Here's how the part is built. I have some questions about the finished solid (model axes, mm). Face numbers are marked on the shaded views. A direction names the side the tool comes from. Give positions to 0.01 mm unless a question says otherwise; leave off trailing zeros. Loops run counter-clockwise (first coordinate to the right, second up) from the corner with the lowest first, then second, coordinate; pieces in that order, holes last.
Q1. Suppose I cut it at A-A (x = 0). List the corners of the cut face in (y, z) for me.
Q2. For the marked faces 1 and 2, which set-ups out of +Z, -Z, +X, -X, +Y, -Y let a thin tool reach every point of the face, with its end or its side?
Q3. I need wall thicknesses on probe 1 along Y at (x, z) = (-10.5, 215); probe 2 along Y at (x, z) = (0, 220.5). Which ranges of each line are inside material? Lowest first, please.
Q4. Thinking about a two-plate mould opening in X: for the marked faces 3, 4, 5 and 6, which applies, pulls with the +X half, pulls with the -X half, needs draft (parallel to the pull), parting line crosses it, or undercut?
Q5. Suppose I cut it at B-B (y = -11.75). List the corners of the cut face in (x, z) for me, and give its area (3 significant figures).
Q6. I'm going to push flat-ended pins straight in: P1, Ø4.5, axis at y = -1, z = 220.5, coming from the +X side; P2, Ø0.7, axis at x = -4.5, z = 214.5, coming from the -Y side; P3, Ø0.6, axis at y = 14.5, z = 228.5, coming from the -X side. Where does each tip first touch, or does it pass through?
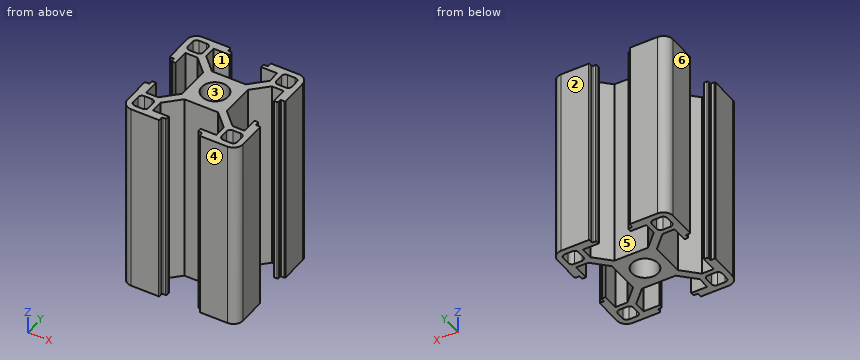
```python
from build123d import *

# Parameters (mm, degrees)
BOSS_EXTRUDE1_DEPTH = 250
SKETCH2_R           = 3.4
CUT_EXTRUDE1_DEPTH  = 251.898385806
FILLET1_R           = 2.5
FILLET2_R           = 0.25
CUT_EXTRUDE3_START  = -200
SKETCH3_R           = 3.4
CUT_EXTRUDE3_DEPTH  = 200


with BuildPart() as part:
    # Sketch1 → Boss-Extrude1 (new body)
    with BuildSketch(Plane.XY):
        Polygon((-15, 15), (-5.2, 15), (-5.2, 13.808325472), (-4.1, 13.808325472), (-4.1, 12.8), (-8.25, 12.8), (-8.25, 9.664213562), (-4.385786438, 5.8), (4.385786438, 5.8), (8.25, 9.664213562), (8.25, 12.8), (4.1, 12.8), (4.1, 13.808325472), (5.2, 13.808325472), (5.2, 15), (15, 15), (15, 5.2), (13.808325472, 5.2), (13.808325472, 4.1), (12.8, 4.1), (12.8, 8.25), (9.664213562, 8.25), (5.8, 4.385786438), (5.8, -4.385786438), (9.664213562, -8.25), (12.8, -8.25), (12.8, -4.1), (13.808325472, -4.1), (13.808325472, -5.2), (15, -5.2), (15, -15), (5.2, -15), (5.2, -13.808325472), (4.1, -13.808325472), (4.1, -12.8), (8.25, -12.8), (8.25, -9.664213562), (4.385786438, -5.8), (-4.385786438, -5.8), (-8.25, -9.664213562), (-8.25, -12.8), (-4.1, -12.8), (-4.1, -13.808325472), (-5.2, -13.808325472), (-5.2, -15), (-15, -15), (-15, -5.2), (-13.808325472, -5.2), (-13.808325472, -4.1), (-12.8, -4.1), (-12.8, -8.25), (-9.664213562, -8.25), (-5.8, -4.385786438), (-5.8, 4.385786438), (-9.664213562, 8.25), (-12.8, 8.25), (-12.8, 4.1), (-13.808325472, 4.1), (-13.808325472, 5.2), (-15, 5.2), align=None)
    extrude(amount=BOSS_EXTRUDE1_DEPTH)

    # Sketch2 → Cut-Extrude1 (cut, through all)
    with BuildSketch(Plane.XY.offset(250)):
        Circle(SKETCH2_R)
        with BuildLine():
            Line((-12.5, 13.5), (-10.5, 13.5))
            ThreePointArc((-10.5, 13.5), (-9.792893219, 13.207106781), (-9.5, 12.5))
            Line((-9.5, 12.5), (-9.5, 10.5))
            ThreePointArc((-9.5, 10.5), (-9.792893219, 9.792893219), (-10.5, 9.5))
            Line((-10.5, 9.5), (-12.5, 9.5))
            ThreePointArc((-12.5, 9.5), (-13.207106781, 9.792893219), (-13.5, 10.5))
            Line((-13.5, 10.5), (-13.5, 12.5))
            ThreePointArc((-13.5, 12.5), (-13.207106781, 13.207106781), (-12.5, 13.5))
        make_face()
        with BuildLine():
            Line((9.5, 12.5), (9.5, 10.5))
            ThreePointArc((9.5, 10.5), (9.792893219, 9.792893219), (10.5, 9.5))
            Line((10.5, 9.5), (12.5, 9.5))
            ThreePointArc((12.5, 9.5), (13.207106781, 9.792893219), (13.5, 10.5))
            Line((13.5, 10.5), (13.5, 12.5))
            ThreePointArc((13.5, 12.5), (13.207106781, 13.207106781), (12.5, 13.5))
            Line((12.5, 13.5), (10.5, 13.5))
            ThreePointArc((10.5, 13.5), (9.792893219, 13.207106781), (9.5, 12.5))
        make_face()
        with BuildLine():
            Line((12.5, -13.5), (10.5, -13.5))
            ThreePointArc((10.5, -13.5), (9.792893219, -13.207106781), (9.5, -12.5))
            Line((9.5, -12.5), (9.5, -10.5))
            ThreePointArc((9.5, -10.5), (9.792893219, -9.792893219), (10.5, -9.5))
            Line((10.5, -9.5), (12.5, -9.5))
            ThreePointArc((12.5, -9.5), (13.207106781, -9.792893219), (13.5, -10.5))
            Line((13.5, -10.5), (13.5, -12.5))
            ThreePointArc((13.5, -12.5), (13.207106781, -13.207106781), (12.5, -13.5))
        make_face()
        with BuildLine():
            Line((-9.5, -12.5), (-9.5, -10.5))
            ThreePointArc((-9.5, -10.5), (-9.792893219, -9.792893219), (-10.5, -9.5))
            Line((-10.5, -9.5), (-12.5, -9.5))
            ThreePointArc((-12.5, -9.5), (-13.207106781, -9.792893219), (-13.5, -10.5))
            Line((-13.5, -10.5), (-13.5, -12.5))
            ThreePointArc((-13.5, -12.5), (-13.207106781, -13.207106781), (-12.5, -13.5))
            Line((-12.5, -13.5), (-10.5, -13.5))
            ThreePointArc((-10.5, -13.5), (-9.792893219, -13.207106781), (-9.5, -12.5))
        make_face()
    extrude(amount=-CUT_EXTRUDE1_DEPTH, mode=Mode.SUBTRACT)

    # Fillet1
    fillet1_edges = [part.edges().sort_by_distance(p)[0] for p in [
        (15, -15, 125),
        (-15, -15, 125),
        (-15, 15, 125),
        (15, 15, 125),
    ]]
    fillet(fillet1_edges, radius=FILLET1_R)

    # Fillet2
    fillet2_edges = [part.edges().sort_by_distance(p)[0] for p in [
        (5.2, -15, 125),
        (5.2, -13.808325472, 125),
        (4.1, -13.808325472, 125),
        (-4.1, -13.808325472, 125),
        (-5.2, -13.808325472, 125),
        (-5.2, -15, 125),
        (-15, -5.2, 125),
        (-13.808325472, -5.2, 125),
        (-13.808325472, -4.1, 125),
        (-13.808325472, 4.1, 125),
        (-13.808325472, 5.2, 125),
        (-15, 5.2, 125),
        (-5.2, 15, 125),
        (-5.2, 13.808325472, 125),
        (-4.1, 13.808325472, 125),
        (4.1, 13.808325472, 125),
        (5.2, 13.808325472, 125),
        (5.2, 15, 125),
        (15, 5.2, 125),
        (13.808325472, 5.2, 125),
        (13.808325472, 4.1, 125),
        (13.808325472, -4.1, 125),
        (13.808325472, -5.2, 125),
        (15, -5.2, 125),
    ]]
    fillet(fillet2_edges, radius=FILLET2_R)

    # Sketch3 → Cut-Extrude3 (cut)
    with BuildSketch(Plane(origin=(0, 0, 0), x_dir=(-1, 0, 0), z_dir=(0, 0, -1)).offset(CUT_EXTRUDE3_START)):
        with BuildLine():
            Line((12.8, 4.1), (13.558325472, 4.1))
            ThreePointArc((13.558325472, 4.1), (13.735102167, 4.173223305), (13.808325472, 4.35))
            Line((13.808325472, 4.35), (13.808325472, 4.95))
            ThreePointArc((13.808325472, 4.95), (13.881548777, 5.126776695), (14.058325472, 5.2))
            Line((14.058325472, 5.2), (14.75, 5.2))
            ThreePointArc((14.75, 5.2), (14.926776695, 5.273223305), (15, 5.45))
            Line((15, 5.45), (15, 12.5))
            ThreePointArc((15, 12.5), (14.267766953, 14.267766953), (12.5, 15))
            Line((12.5, 15), (5.45, 15))
            ThreePointArc((5.45, 15), (5.273223305, 14.926776695), (5.2, 14.75))
            Line((5.2, 14.75), (5.2, 14.058325472))
            ThreePointArc((5.2, 14.058325472), (5.126776695, 13.881548777), (4.95, 13.808325472))
            Line((4.95, 13.808325472), (4.35, 13.808325472))
            ThreePointArc((4.35, 13.808325472), (4.173223305, 13.735102167), (4.1, 13.558325472))
            Line((4.1, 13.558325472), (4.1, 12.8))
            Line((4.1, 12.8), (8.25, 12.8))
            Line((8.25, 12.8), (8.25, 9.664213562))
            Line((8.25, 9.664213562), (4.385786438, 5.8))
            Line((4.385786438, 5.8), (-4.385786438, 5.8))
            Line((-4.385786438, 5.8), (-8.25, 9.664213562))
            Line((-8.25, 9.664213562), (-8.25, 12.8))
            Line((-8.25, 12.8), (-4.1, 12.8))
            Line((-4.1, 12.8), (-4.1, 13.558325472))
            ThreePointArc((-4.1, 13.558325472), (-4.173223305, 13.735102167), (-4.35, 13.808325472))
            Line((-4.35, 13.808325472), (-4.95, 13.808325472))
            ThreePointArc((-4.95, 13.808325472), (-5.126776695, 13.881548777), (-5.2, 14.058325472))
            Line((-5.2, 14.058325472), (-5.2, 14.75))
            ThreePointArc((-5.2, 14.75), (-5.273223305, 14.926776695), (-5.45, 15))
            Line((-5.45, 15), (-12.5, 15))
            ThreePointArc((-12.5, 15), (-14.267766953, 14.267766953), (-15, 12.5))
            Line((-15, 12.5), (-15, 5.45))
            ThreePointArc((-15, 5.45), (-14.926776695, 5.273223305), (-14.75, 5.2))
            Line((-14.75, 5.2), (-14.058325472, 5.2))
            ThreePointArc((-14.058325472, 5.2), (-13.881548777, 5.126776695), (-13.808325472, 4.95))
            Line((-13.808325472, 4.95), (-13.808325472, 4.35))
            ThreePointArc((-13.808325472, 4.35), (-13.735102167, 4.173223305), (-13.558325472, 4.1))
            Line((-13.558325472, 4.1), (-12.8, 4.1))
            Line((-12.8, 4.1), (-12.8, 8.25))
            Line((-12.8, 8.25), (-9.664213562, 8.25))
            Line((-9.664213562, 8.25), (-5.8, 4.385786438))
            Line((-5.8, 4.385786438), (-5.8, -4.385786438))
            Line((-5.8, -4.385786438), (-9.664213562, -8.25))
            Line((-9.664213562, -8.25), (-12.8, -8.25))
            Line((-12.8, -8.25), (-12.8, -4.1))
            Line((-12.8, -4.1), (-13.558325472, -4.1))
            ThreePointArc((-13.558325472, -4.1), (-13.735102167, -4.173223305), (-13.808325472, -4.35))
            Line((-13.808325472, -4.35), (-13.808325472, -4.95))
            ThreePointArc((-13.808325472, -4.95), (-13.881548777, -5.126776695), (-14.058325472, -5.2))
            Line((-14.058325472, -5.2), (-14.75, -5.2))
            ThreePointArc((-14.75, -5.2), (-14.926776695, -5.273223305), (-15, -5.45))
            Line((-15, -5.45), (-15, -12.5))
            ThreePointArc((-15, -12.5), (-14.267766953, -14.267766953), (-12.5, -15))
            Line((-12.5, -15), (-5.45, -15))
            ThreePointArc((-5.45, -15), (-5.273223305, -14.926776695), (-5.2, -14.75))
            Line((-5.2, -14.75), (-5.2, -14.058325472))
            ThreePointArc((-5.2, -14.058325472), (-5.126776695, -13.881548777), (-4.95, -13.808325472))
            Line((-4.95, -13.808325472), (-4.35, -13.808325472))
            ThreePointArc((-4.35, -13.808325472), (-4.173223305, -13.735102167), (-4.1, -13.558325472))
            Line((-4.1, -13.558325472), (-4.1, -12.8))
            Line((-4.1, -12.8), (-8.25, -12.8))
            Line((-8.25, -12.8), (-8.25, -9.664213562))
            Line((-8.25, -9.664213562), (-4.385786438, -5.8))
            Line((-4.385786438, -5.8), (4.385786438, -5.8))
            Line((4.385786438, -5.8), (8.25, -9.664213562))
            Line((8.25, -9.664213562), (8.25, -12.8))
            Line((8.25, -12.8), (4.1, -12.8))
            Line((4.1, -12.8), (4.1, -13.558325472))
            ThreePointArc((4.1, -13.558325472), (4.173223305, -13.735102167), (4.35, -13.808325472))
            Line((4.35, -13.808325472), (4.95, -13.808325472))
            ThreePointArc((4.95, -13.808325472), (5.126776695, -13.881548777), (5.2, -14.058325472))
            Line((5.2, -14.058325472), (5.2, -14.75))
            ThreePointArc((5.2, -14.75), (5.273223305, -14.926776695), (5.45, -15))
            Line((5.45, -15), (12.5, -15))
            ThreePointArc((12.5, -15), (14.267766953, -14.267766953), (15, -12.5))
            Line((15, -12.5), (15, -5.45))
            ThreePointArc((15, -5.45), (14.926776695, -5.273223305), (14.75, -5.2))
            Line((14.75, -5.2), (14.058325472, -5.2))
            ThreePointArc((14.058325472, -5.2), (13.881548777, -5.126776695), (13.808325472, -4.95))
            Line((13.808325472, -4.95), (13.808325472, -4.35))
            ThreePointArc((13.808325472, -4.35), (13.735102167, -4.173223305), (13.558325472, -4.1))
            Line((13.558325472, -4.1), (12.8, -4.1))
            Line((12.8, -4.1), (12.8, -8.25))
            Line((12.8, -8.25), (9.664213562, -8.25))
            Line((9.664213562, -8.25), (5.8, -4.385786438))
            Line((5.8, -4.385786438), (5.8, 4.385786438))
            Line((5.8, 4.385786438), (9.664213562, 8.25))
            Line((9.664213562, 8.25), (12.8, 8.25))
            Line((12.8, 8.25), (12.8, 4.1))
        make_face()
        with Locations(Location((0, 0, 0), (0, 0, 180))):
            Circle(SKETCH3_R, mode=Mode.SUBTRACT)
        with BuildLine():
            Line((-9.5, 12.5), (-9.5, 10.5))
            ThreePointArc((-9.5, 10.5), (-9.792893219, 9.792893219), (-10.5, 9.5))
            Line((-10.5, 9.5), (-12.5, 9.5))
            ThreePointArc((-12.5, 9.5), (-13.207106781, 9.792893219), (-13.5, 10.5))
            Line((-13.5, 10.5), (-13.5, 12.5))
            ThreePointArc((-13.5, 12.5), (-13.207106781, 13.207106781), (-12.5, 13.5))
            Line((-12.5, 13.5), (-10.5, 13.5))
            ThreePointArc((-10.5, 13.5), (-9.792893219, 13.207106781), (-9.5, 12.5))
        make_face(mode=Mode.SUBTRACT)
        with BuildLine():
            Line((12.5, 9.5), (10.5, 9.5))
            ThreePointArc((10.5, 9.5), (9.792893219, 9.792893219), (9.5, 10.5))
            Line((9.5, 10.5), (9.5, 12.5))
            ThreePointArc((9.5, 12.5), (9.792893219, 13.207106781), (10.5, 13.5))
            Line((10.5, 13.5), (12.5, 13.5))
            ThreePointArc((12.5, 13.5), (13.207106781, 13.207106781), (13.5, 12.5))
            Line((13.5, 12.5), (13.5, 10.5))
            ThreePointArc((13.5, 10.5), (13.207106781, 9.792893219), (12.5, 9.5))
        make_face(mode=Mode.SUBTRACT)
        with BuildLine():
            Line((9.5, -12.5), (9.5, -10.5))
            ThreePointArc((9.5, -10.5), (9.792893219, -9.792893219), (10.5, -9.5))
            Line((10.5, -9.5), (12.5, -9.5))
            ThreePointArc((12.5, -9.5), (13.207106781, -9.792893219), (13.5, -10.5))
            Line((13.5, -10.5), (13.5, -12.5))
            ThreePointArc((13.5, -12.5), (13.207106781, -13.207106781), (12.5, -13.5))
            Line((12.5, -13.5), (10.5, -13.5))
            ThreePointArc((10.5, -13.5), (9.792893219, -13.207106781), (9.5, -12.5))
        make_face(mode=Mode.SUBTRACT)
        with BuildLine():
            Line((-9.5, -10.5), (-9.5, -12.5))
            ThreePointArc((-9.5, -12.5), (-9.792893219, -13.207106781), (-10.5, -13.5))
            Line((-10.5, -13.5), (-12.5, -13.5))
            ThreePointArc((-12.5, -13.5), (-13.207106781, -13.207106781), (-13.5, -12.5))
            Line((-13.5, -12.5), (-13.5, -10.5))
            ThreePointArc((-13.5, -10.5), (-13.207106781, -9.792893219), (-12.5, -9.5))
            Line((-12.5, -9.5), (-10.5, -9.5))
            ThreePointArc((-10.5, -9.5), (-9.792893219, -9.792893219), (-9.5, -10.5))
        make_face(mode=Mode.SUBTRACT)
    extrude(amount=CUT_EXTRUDE3_DEPTH, mode=Mode.SUBTRACT)


solid = part.part
```
Solutions:
1. outline: (-5.8, 200) - (-3.4, 200) - (-3.4, 250) - (-5.8, 250) - close; (3.4, 200) - (5.8, 200) - (5.8, 250) - (3.4, 250) - close
2. face 1: +Z, -Z
2. face 2: +Z, -Z, +X, -X, +Y
3. probe 1: y = -15 to -13.5, -9.5 to -8.25, 8.25 to 9.5, 13.5 to 15
3. probe 2: y = -5.8 to -3.4, 3.4 to 5.8
4. face 3: undercut
4. face 4: needs draft
4. face 5: undercut
4. face 6: pulls with the -X half
5. outline: (-15, 200) - (-13.5, 200) - (-13.5, 250) - (-15, 250) - close; (-9.5, 200) - (-8.25, 200) - (-8.25, 250) - (-9.5, 250) - close; (8.25, 200) - (9.5, 200) - (9.5, 250) - (8.25, 250) - close; (13.5, 200) - (15, 200) - (15, 250) - (13.5, 250) - close
5. area: 275 mm2
6. P1: stops at x = 5.8
6. P2: stops at y = -13.81
6. P3: stops at x = -14.33
